Verification items for the finished model (mm, model axes). A direction names the side the tool comes from. Give positions to 0.01 mm unless a question says otherwise; leave off trailing zeros. Loops run counter-clockwise (first coordinate to the right, second up) from the corner with the lowest first, then second, coordinate; pieces in that order, holes last. Notation, with made-up numbers: M 67,39 L 104,39 A29 cw 104,62 Z; hole C -2,-26.5 d9. An arc over 180 degrees is marked long. Use CSV: the item, a comma, the result in double quotes.
from build123d import *

# Parameters (mm, degrees)
SKETCH_1_W                 = 2.5
SKETCH_1_H                 = 40
SKETCH_8_R                 = 1.45
EXTRUDE_2_DEPTH            = 5
PATTERN_CIRCULAR_760_COUNT = 3
EXTRUDE_2_2_DEPTH          = 20
EXTRUDE_2_2_DEPTH_BACK     = 40
SKETCH_5_R                 = 2.5
SKETCH_6_R                 = 1
EXTRUDE_1_DEPTH            = 40
PATTERN_CIRCULAR_1_COUNT   = 3
SKETCH_9_R                 = 1.45
EXTRUDE_3_DEPTH            = 5


with BuildPart() as part:
    # 草图1 → 杆件1 (revolve)
    with BuildSketch(Plane(origin=(0, 0, 0), x_dir=(1, 0, 0), z_dir=(0, 1, 0)), mode=Mode.PRIVATE) as revolve_1_sk:
        with Locations((-1.25, 20)):
            Rectangle(SKETCH_1_W, SKETCH_1_H)
    revolve_1 = revolve(revolve_1_sk.sketch.rotate(Axis((0, 0, 0), (0, 0, -1)), 180), axis=Axis((0, 0, 0), (0, 0, -1)))

    # 草图8 → Extrude 2 (add)
    with BuildSketch(Plane(origin=(0, 0, -40), x_dir=(-1, 0, 0), z_dir=(0, 0, -1))):
        Circle(SKETCH_8_R)
    extrude_2 = extrude(amount=EXTRUDE_2_DEPTH)

    # Pattern Circular 760: 杆件1 ×3 about axis
    pattern_circular_760_axis = Axis((0, 0, 0), (0, 1, 0))
    for i in range(1, PATTERN_CIRCULAR_760_COUNT):
        add(revolve_1.rotate(pattern_circular_760_axis, i * 360 / PATTERN_CIRCULAR_760_COUNT))

    # 草图5 → Extrude 2 2 (add, two sides: drawn at the far end of the back side and taken through both)
    with BuildSketch(Plane(origin=(0, 0, 0), x_dir=(1, 0, 0), z_dir=(0, 1, 0)).offset(-EXTRUDE_2_2_DEPTH_BACK)):
        with Locations(Location((0, 0, 0), (0, 0, 270))):
            Circle(SKETCH_5_R)
    extrude(amount=EXTRUDE_2_2_DEPTH + EXTRUDE_2_2_DEPTH_BACK)

    # 草图6 → 凸台-拉伸1 (add)
    with BuildSketch(Plane(origin=(0, 20, 0), x_dir=(1, 0, 0), z_dir=(0, 1, 0))):
        with Locations(Location((0, 0, 0), (0, 0, 270))):
            Circle(SKETCH_6_R)
    extrude(amount=EXTRUDE_1_DEPTH)

    # 阵列(圆周)1: Extrude 2 ×3 about axis
    pattern_circular_1_axis = Axis((0, 0, 0), (0, 1, 0))
    for i in range(1, PATTERN_CIRCULAR_1_COUNT):
        add(extrude_2.rotate(pattern_circular_1_axis, i * 360 / PATTERN_CIRCULAR_1_COUNT))

    # 草图9 → 凸台-拉伸3 (add)
    with BuildSketch(Plane.XZ.offset(40)):
        with Locations(Location((0, 0, 0), (0, 0, 270))):
            Circle(SKETCH_9_R)
    extrude(amount=EXTRUDE_3_DEPTH)


solid = part.part
(1) Tool access check on faces 1 (the flat face through (-34.624, 1.632, 20.03)), 2 (the cylindrical face through (-2.5, -0.1, -20.9)), 3 (the flat face through (-2, -40, 0)), 4 (the flat face through (-38.981, 0.02, 22.482)), 5 (the cylindrical face through (0.751, 10.494, 2.385)). Record the directions out of +Z, -Z, +X, -X, +Y, -Y that give a thin tool (end or side, any length) a straight path to the whole face; none if there is none.
Calculated:
face 1,"none"
face 2,"-Z"
face 3,"-Y"
face 4,"+Z, -X, +Y, -Y"
face 5,"+Y"
(2) Mould release check, pull along X, two halves, no side actions. Record for faces 6 (the cylindrical face through (0.06, -42.46, 1.45)), 7 (the flat face through (2, 0, -40)), 8 (the flat face through (33.825, -0.035, 21.413)): released by +X, released by -X, zero draft, split by the parting line, or undercut.
Calculated:
face 6,"split by the parting line"
face 7,"zero draft"
face 8,"undercut"
(3) Depth check by flat-ended pin: pin 1 Ø10 at (x, z) = (5.5, -17) entering from +Y; pin 2 Ø12 at (x, y) = (19.5, 12) entering from -Z; pin 3 Ø3 at (x, z) = (-0.5, -31.5) entering from -Y. Enter the tip coordinate at first touch or a pass-through.
Calculated:
pin 1,"stops at y = 2.45"
pin 2,"passes through"
pin 3,"stops at y = -2.5"
(4) Scan lines: L1, parallel to Y at x = -1, z = -7.5; L2, parallel to Y at x = -0.5, z = -36. Record each from-to range of solid material in increasing order. Write a range as from..to.
Calculated:
L1,"y = -2.29..2.29"
L2,"y = -2.45..2.45"
(5) Section check B-B on z = -28. Record the cut outline in (x, y), plus the area to 3 significant figures.
Calculated:
outline,"C 0,0 d5"
area,"19.6 mm²"
(6) Section check A-A on y = 39. Record the cut outline in (x, z), plus the area to 3 significant figures.
Calculated:
outline,"C 0,0 d2"
area,"3.14 mm²"
(7) Section check C-C on y = 0. Record the cut outline in (x, z), plus the area to 3 significant figures.
Calculated:
outline,"M -39.7,21.24 L -35.37,18.74 L -35.89,17.83 L -2.5,-1.44 L -2.5,-40 L -1.45,-40 L -1.45,-45 L 1.45,-45 L 1.45,-40 L 2.5,-40 L 2.5,-1.44 L 35.89,17.83 L 35.37,18.74 L 39.7,21.24 L 38.25,23.76 L 33.92,21.26 L 33.39,22.17 L 0,2.89 L -33.39,22.17 L -33.92,21.26 L -38.25,23.76 Z"
area,"633 mm²"
